CAD build for the part. Positions are in the model's coordinates, mm. Face numbers are marked on the shaded views. A direction names the side the tool comes from. Give positions to 0.01 mm unless a question says otherwise; leave off trailing zeros. Order: outer loops, then holes, each group sorted by start corner. A loop starts at its lowest first (then second) coordinate and runs counter-clockwise, first axis right, second up. Notation, with made-up numbers: (40.5, 59) -> (66.5, 59) arc R32 ccw to (66.5, 92) -> close; hole circle Ø4 at (58.25, 57). An arc over 180 degrees is marked (long way). Use one line per item in the form item = value. Start each with the question number.
1) Drop flat-ended pins along their axis: P1, Ø5, axis at x = 4.5, z = 12, coming from the +Y side; P2, Ø1.5, axis at y = -3, z = 24.5, coming from the -X side; P3, Ø1, axis at y = 4, z = 4, coming from the -X side; P4, Ø6, axis at x = 8.5, y = -0.5, coming from the +Z side. Give the stop position or say it passes through.
2) Cut at C-C, the plane z = 20.25. Give the cut face in (x, y) (3 decimals).
3) Mould opens along Y. For the marked faces 3, 4, 5 and 6 say: pulls with the +Y half, pulls with the -Y half, needs draft (parallel to the pull), parting line crosses it, or undercut.
4) Cut at A-A, the plane y = 0. Give the cut face in (x, z) (1 decimal), and give its area (3 significant figures).
5) Probe line 1 (Y direction, x = 0, z = 23.5) (3 decimals); line 2 (Y direction, x = 0, z = 7.5); line 3 (Z direction, x = 5.25, y = 5.25). List the from-to ranges inside material, lowest first.
6) Cut at B-B, the plane x = -1.5. Give the cut face in (y, z), and give its area (3 significant figures).
7) Cut at D-D, the plane y = 2.5. Give the cut face in (x, z).
8) Tool access for the marked faces 1 and 2: list every direction of +Z, -Z, +X, -X, +Y, -Y with a clear straight run to the whole face (end or side of a thin tool).
from build123d import *

# Parameters (mm, degrees)
F0_R     = 10.4775
F1_DEPTH = 13.97
F2_R     = 7.366
F3_DEPTH = 14.986
F4_R     = 8.5979
F5_DEPTH = 11.43
F6_R     = 1.905
F7_DEPTH = 17.78


with BuildPart() as f1:
    # F0 (on Top) → F1 (new body)
    with BuildSketch(Plane.XY):
        Circle(F0_R)
    extrude(amount=F1_DEPTH)

    # F2 (on face) → F3 (join)
    with BuildSketch(Plane.XY.offset(13.97)):
        Circle(F2_R)
    extrude(amount=F3_DEPTH)

    # F4 (on face) → F5 (cut)
    with BuildSketch(Plane(origin=(0, 0, 0), x_dir=(1, 0, 0), z_dir=(0, 0, -1))):
        Circle(F4_R)
    extrude(amount=-F5_DEPTH, mode=Mode.SUBTRACT)

    # F6 (on face) → F7 (cut)
    with BuildSketch(Plane(origin=(0, 0, 11.43), x_dir=(1, 0, 0), z_dir=(0, 0, -1))):
        Circle(F6_R)
    extrude(amount=-F7_DEPTH, mode=Mode.SUBTRACT)


solid = f1.part
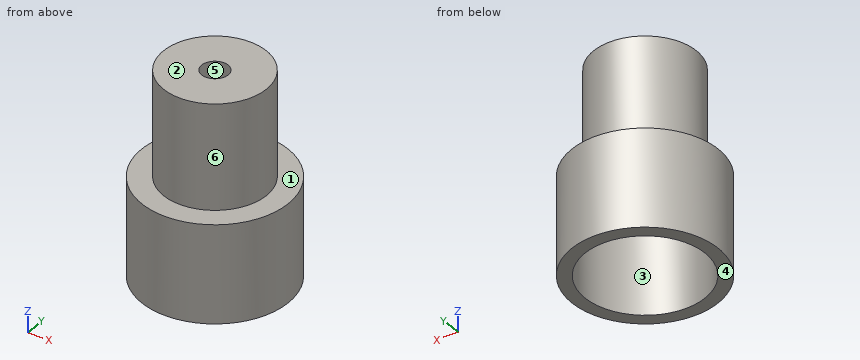
Result:
q1.P1 = 10.28
q1.P2 = -7.01
q1.P3 = -9.88
q1.P4 = 28.96
q2.outline = circle Ø14.732 at (0, 0); hole circle Ø3.81 at (0, 0)
q3.face_3 = undercut
q3.face_4 = needs draft
q3.face_5 = undercut
q3.face_6 = parting line crosses it
q4.outline = (-10.5, 0) -> (-8.6, 0) -> (-8.6, 11.4) -> (-1.9, 11.4) -> (-1.9, 29) -> (-7.4, 29) -> (-7.4, 14) -> (-10.5, 14) -> close; (1.9, 11.4) -> (8.6, 11.4) -> (8.6, 0) -> (10.5, 0) -> (10.5, 14) -> (7.4, 14) -> (7.4, 29) -> (1.9, 29) -> close
q4.area = 250 mm²
q5.line_1 = -7.366 to -1.905, 1.905 to 7.366
q5.line_2 = -10.48 to -8.6, 8.6 to 10.48
q5.line_3 = 11.43 to 13.97
q6.outline = (-10.37, 0) -> (-8.47, 0) -> (-8.47, 11.43) -> (-1.17, 11.43) -> (-1.17, 28.96) -> (-7.21, 28.96) -> (-7.21, 13.97) -> (-10.37, 13.97) -> close; (1.17, 11.43) -> (8.47, 11.43) -> (8.47, 0) -> (10.37, 0) -> (10.37, 13.97) -> (7.21, 13.97) -> (7.21, 28.96) -> (1.17, 28.96) -> close
q6.area = 271 mm²
q7.outline = (-10.17, 0) -> (-8.23, 0) -> (-8.23, 11.43) -> (8.23, 11.43) -> (8.23, 0) -> (10.17, 0) -> (10.17, 13.97) -> (6.93, 13.97) -> (6.93, 28.96) -> (-6.93, 28.96) -> (-6.93, 13.97) -> (-10.17, 13.97) -> close
q8.face_1 = +Z
q8.face_2 = +Z, +X, -X, +Y, -Y
